Input: part model. Units: mm. Frame: model coordinates. A direction names the side the tool comes from. Coordinates: 2 decimals unless noted, no trailing zeros. Order: outer loops, then holes, each group sorted by start corner. A loop starts at its lowest first (then second) coordinate and runs counter-clockwise, first axis right, second up.
from build123d import *

# Parameters (mm, degrees)
P_IDAT_VYSUNUT_M1_DEPTH  = 50
ZKOSEN_1_SIZE            = 40
ZKOSEN_2_SIZE            = 40
SKICA2_R                 = 1.65
ODEBRAT_VYSUNUT_M1_DEPTH = 37
ZAOBLIT1_R               = 5
ODEBRAT_VYSUNUT_M2_DEPTH = 2.5
ODEBRAT_VYSUNUT_M3_DEPTH = 2.5
SKICA7_R                 = 1.65
ODEBRAT_VYSUNUT_M4_DEPTH = 56
ODEBRAT_VYSUNUT_M5_DEPTH = 2.5


with BuildPart() as part:
    # Skica1 → Přidat vysunutím1 (new body)
    with BuildSketch(Plane.XY):
        Polygon((0, 0), (0, 55), (8, 55), (8, 7), (28, 7), (28, 55), (36, 55), (36, 0), align=None)
    extrude(amount=P_IDAT_VYSUNUT_M1_DEPTH)

    # Zkosení1
    zkosen_1_edges = [part.edges().sort_by_distance(p)[0] for p in [
        (32, 55, 50),
    ]]
    chamfer(zkosen_1_edges, length=ZKOSEN_1_SIZE)

    # Zkosení2
    zkosen_2_edges = [part.edges().sort_by_distance(p)[0] for p in [
        (4, 55, 50),
    ]]
    chamfer(zkosen_2_edges, length=ZKOSEN_2_SIZE)

    # Skica2 → Odebrat vysunutím1 (cut, through all)
    with BuildSketch(Plane(origin=(36, 0, 0), x_dir=(0, 0, -1), z_dir=(1, 0, 0))):
        with Locations((-5, 50)):
            Circle(SKICA2_R)
        with Locations((-5, 10)):
            Circle(SKICA2_R)
        with Locations((-25, 20)):
            Circle(SKICA2_R)
    extrude(amount=-ODEBRAT_VYSUNUT_M1_DEPTH, mode=Mode.SUBTRACT)

    # Zaoblit1
    zaoblit1_edges = [part.edges().sort_by_distance(p)[0] for p in [
        (32, 15, 50),
        (32, 55, 10),
        (4, 15, 50),
        (4, 55, 10),
        (4, 55, 0),
        (32, 55, 0),
    ]]
    fillet(zaoblit1_edges, radius=ZAOBLIT1_R)

    # Skica3 → Odebrat vysunutím2 (cut)
    with BuildSketch(Plane.ZY.offset(-28)):
        Polygon((6.58771324, 52.75), (3.41228676, 52.75), (1.824573519, 50), (3.41228676, 47.25), (6.58771324, 47.25), (8.175426481, 50), align=None)
        Polygon((6.58771324, 12.75), (3.41228676, 12.75), (1.824573519, 10), (3.41228676, 7.25), (6.58771324, 7.25), (8.175426481, 10), align=None)
    extrude(amount=-ODEBRAT_VYSUNUT_M2_DEPTH, mode=Mode.SUBTRACT)

    # Skica6 → Odebrat vysunutím3 (cut)
    with BuildSketch(Plane(origin=(8, 0, 0), x_dir=(0, 0, -1), z_dir=(1, 0, 0))):
        Polygon((-3.41228676, 52.75), (-6.58771324, 52.75), (-8.175426481, 50), (-6.58771324, 47.25), (-3.41228676, 47.25), (-1.824573519, 50), align=None)
        Polygon((-3.41228676, 12.75), (-6.58771324, 12.75), (-8.175426481, 10), (-6.58771324, 7.25), (-3.41228676, 7.25), (-1.824573519, 10), align=None)
    extrude(amount=-ODEBRAT_VYSUNUT_M3_DEPTH, mode=Mode.SUBTRACT)

    # Skica7 → Odebrat vysunutím4 (cut, through all)
    with BuildSketch(Plane.XZ):
        with Locations((18, 44.5)):
            Circle(SKICA7_R)
        with Locations((18, 25.45)):
            Circle(SKICA7_R)
        with Locations((18, 6.4)):
            Circle(SKICA7_R)
    extrude(amount=-ODEBRAT_VYSUNUT_M4_DEPTH, mode=Mode.SUBTRACT)

    # Skica8 → Odebrat vysunutím5 (cut)
    with BuildSketch(Plane(origin=(0, 7, 0), x_dir=(1, 0, 0), z_dir=(0, 1, 0))):
        Polygon((14.824573519, -6.4), (16.41228676, -9.15), (19.58771324, -9.15), (21.175426481, -6.4), (19.58771324, -3.65), (16.41228676, -3.65), align=None)
        Polygon((14.824573519, -25.45), (16.41228676, -28.2), (19.58771324, -28.2), (21.175426481, -25.45), (19.58771324, -22.7), (16.41228676, -22.7), align=None)
        Polygon((14.824573519, -44.5), (16.41228676, -47.25), (19.58771324, -47.25), (21.175426481, -44.5), (19.58771324, -41.75), (16.41228676, -41.75), align=None)
    extrude(amount=-ODEBRAT_VYSUNUT_M5_DEPTH, mode=Mode.SUBTRACT)


solid = part.part
Item 1: Draft query along Y for faces 6 (the face through (4.056, 21.115, 26.216)), 7 (the face through (19.4, 4.5, 5.1)), 8 (the face through (14, 0, 25)). Return one class per face: pulls with the +Y half, pulls with the -Y half, needs draft (parallel to the pull), parting line crosses it, or undercut.
Response values:
face 6: undercut
face 7: pulls with the +Y half
face 8: pulls with the -Y half
Item 2: Cut plane D-D on z = 15.5. Return loops of the section in (x, y), then the cut area to 3 significant figures.
Response values:
outline: (0, 0) - (36, 0) - (36, 49.5) - (28, 49.5) - (28, 7) - (8, 7) - (8, 49.5) - (0, 49.5) - close
area: 932 mm2
Item 3: Access query for faces 1 (the face through (18, 5, 50)), 2 (the face through (18, 6, 28.2)), 3 (the face through (32, 35, 30)), 4 (the face through (28, 25, 19)), 5 (the face through (29.23, 48.64, 2.61)). Directions: +Z, -Z, +X, -X, +Y, -Y. A direction counts if a zero-diameter tool reaches every point of the face in a straight line with its end or side. Return the directions, or none.
Response values:
face 1: +Z, +X, -X, +Y, -Y
face 2: +Y
face 3: +Z, +X, -X, +Y
face 4: +Z, -Z, +Y
face 5: none
Item 4: Ray query, probe 1 along X at (y, z) = (16.5, 11.5); probe 2 along X at (y, z) = (1, 44); probe 3 along Y at (x, z) = (34.4, 5). Return the intervals inside material, ascending.
Response values:
probe 1: x = 0 to 8, 28 to 36
probe 2: x = 0 to 16.43, 19.57 to 36
probe 3: y = 0 to 8.35, 11.65 to 48.35, 51.65 to 55
Item 5: Pin query (flat end, axial travel): pin 1 Ø4.5 at (x, z) = (17, 44.5) entering from +Y; pin 2 Ø4 at (x, z) = (31, 39) entering from +Y; pin 3 Ø10 at (x, z) = (8.5, 32) entering from +Y. Return the tip coordinate at first contact, or that it passes through.
Response values:
pin 1: stops at y = 7
pin 2: stops at y = 28
pin 3: stops at y = 37.97
Item 6: Cut plane C-C on y = 45.5. Return loops of the section in (x, z).
Response values:
outline: (0, 0) - (8, 0) - (8, 19.5) - (0, 19.5) - close; (28, 0) - (36, 0) - (36, 19.5) - (28, 19.5) - close
Item 7: Cut plane B-B on x = 31.5. Return loops of the section in (y, z).
Response values:
outline: (0, 0) - (50, 0) arc R5 ccw to (55, 5) - (55, 7.93) arc R5 ccw to (53.54, 11.46) - (16.46, 48.54) arc R5 ccw to (12.93, 50) - (0, 50) - close; hole circle Ø3.3 at (10, 5); hole circle Ø3.3 at (20, 25); hole circle Ø3.3 at (50, 5)
Item 8: Cut plane A-A on y = 20. Return loops of the section in (x, z), then the cut area to 3 significant figures.
Response values:
outline: (0, 0) - (8, 0) - (8, 23.35) - (0, 23.35) - close; (0, 26.65) - (8, 26.65) - (8, 45) - (0, 45) - close; (28, 0) - (36, 0) - (36, 23.35) - (28, 23.35) - close; (28, 26.65) - (36, 26.65) - (36, 45) - (28, 45) - close
area: 667 mm2
